from build123d import *

# Parameters (mm, degrees)
SKETCH_1_W          = 400
SKETCH_1_H          = 90
EXTRUDE_1_DEPTH     = 10
SKETCH_2_R          = 9.063152432
CUT_EXTRUDE_1_DEPTH = 10
SKETCH_3_R          = 1.81023823
SKETCH_3_R_2        = 1.954373085
SKETCH_3_R_3        = 2.399911157
SKETCH_3_R_4        = 2.359906839
CUT_EXTRUDE_2_DEPTH = 10
SKETCH_4_R          = 6.073356137
SKETCH_4_R_2        = 6.104859493
SKETCH_4_R_3        = 4.740379866
CUT_EXTRUDE_3_DEPTH = 10
SKETCH_5_W          = 12.49982796
SKETCH_5_H          = 90
EXTRUDE_2_DEPTH     = 270
SKETCH_6_W          = 148.075925294
SKETCH_6_H          = 90
CUT_EXTRUDE_4_DEPTH = 10
SKETCH_7_W          = 153.736310317
SKETCH_7_H          = 106.42917614
CUT_EXTRUDE_5_DEPTH = 10


with BuildPart() as part:
    # 草图1 → 凸台-拉伸1 (new body)
    with BuildSketch(Plane(origin=(0, 0, 0), x_dir=(1, 0, 0), z_dir=(0, 1, 0))):
        Rectangle(SKETCH_1_W, SKETCH_1_H)
    extrude(amount=EXTRUDE_1_DEPTH)

    # 草图2 → 切除-拉伸1 (cut)
    with BuildSketch(Plane(origin=(0, 10, 0), x_dir=(1, 0, 0), z_dir=(0, 1, 0))):
        with Locations((-6, 0)):
            Circle(SKETCH_2_R)
    extrude(amount=-CUT_EXTRUDE_1_DEPTH, mode=Mode.SUBTRACT)

    # 草图3 → 切除-拉伸2 (cut)
    with BuildSketch(Plane(origin=(0, 10, 0), x_dir=(1, 0, 0), z_dir=(0, 1, 0))):
        with Locations((-6, 25)):
            Circle(SKETCH_3_R)
        with Locations((19, 0)):
            Circle(SKETCH_3_R_2)
        with Locations((-6, -25)):
            Circle(SKETCH_3_R_3)
        with Locations((-31, 0)):
            Circle(SKETCH_3_R_4)
    extrude(amount=-CUT_EXTRUDE_2_DEPTH, mode=Mode.SUBTRACT)

    # 草图4 → 切除-拉伸3 (cut)
    with BuildSketch(Plane(origin=(0, 10, 0), x_dir=(1, 0, 0), z_dir=(0, 1, 0))):
        with Locations((-175, -21.552072621)):
            Circle(SKETCH_4_R)
        with Locations((-135, -21.552072621)):
            Circle(SKETCH_4_R_2)
        with Locations((-155, 23.447927379)):
            Circle(SKETCH_4_R_3)
    extrude(amount=-CUT_EXTRUDE_3_DEPTH, mode=Mode.SUBTRACT)

    # 草图5 → 凸台-拉伸2 (add)
    with BuildSketch(Plane(origin=(0, 10, 0), x_dir=(1, 0, 0), z_dir=(0, 1, 0))):
        with Locations((45.073880923, 0)):
            Rectangle(SKETCH_5_W, SKETCH_5_H)
    extrude(amount=EXTRUDE_2_DEPTH)

    # 草图6 → 切除-拉伸4 (cut)
    with BuildSketch(Plane.XZ):
        with Locations((-125.962037353, 0)):
            Rectangle(SKETCH_6_W, SKETCH_6_H)
    extrude(amount=-CUT_EXTRUDE_4_DEPTH, mode=Mode.SUBTRACT)

    # 草图7 → 切除-拉伸5 (cut)
    with BuildSketch(Plane(origin=(0, 10, 0), x_dir=(1, 0, 0), z_dir=(0, 1, 0))):
        with Locations((128.191950062, -8.21458807)):
            Rectangle(SKETCH_7_W, SKETCH_7_H)
    extrude(amount=-CUT_EXTRUDE_5_DEPTH, mode=Mode.SUBTRACT)


solid = part.part
Read the model definition and answer for the solid it produces. Units are mm, in the model's axes. A direction names the side the tool comes from. Coordinates: 2 decimals unless noted, no trailing zeros. Loops run counter-clockwise (first coordinate to the right, second up) from the corner with the lowest first, then second, coordinate; pieces in that order, holes last. Notation, with made-up numbers: (5, -8) -> (37, -8) arc R33 cw to (37, 27) -> close; hole circle Ø5 at (-33, -38.5). An arc over 180 degrees is marked (long way). Answer in a Markdown table with one row per item.
Item 1: A cutting plane is placed at C-C on y = 228. Determine the outline of the cut face in (x, z), plus the area to 3 significant figures.
Returned:
| item | result |
|---|---|
| outline | (38.82, -45) -> (51.32, -45) -> (51.32, 45) -> (38.82, 45) -> close |
| area | 1,120 mm^2 |
Item 2: Straight lines are drawn through the part: line 1 along Z through (x, y) = (-6, 4); line 2 along X through (y, z) = (8.25, 0); line 3 along Z through (x, y) = (-31, 2.5). For each, find the intervals that lie inside material, in ascending order. Write a range as [from, to].
Returned:
| item | result |
|---|---|
| line 1 | z = [-45, -26.81], [-23.19, -9.06], [9.06, 22.6], [27.4, 45] |
| line 2 | x = [-51.92, -33.36], [-28.64, -15.06], [3.06, 17.05], [20.95, 51.32] |
| line 3 | z = [-45, -2.36], [2.36, 45] |
Item 3: A cutting plane is placed at D-D on x = -22.5. Determine the outline of the cut face in (y, z).
Returned:
| item | result |
|---|---|
| outline | (0, -45) -> (10, -45) -> (10, 45) -> (0, 45) -> close |
Item 4: A cutting plane is placed at A-A on x = -11.5. Determine the outline of the cut face in (y, z).
Returned:
| item | result |
|---|---|
| outline | (0, -45) -> (10, -45) -> (10, -7.2) -> (0, -7.2) -> close; (0, 7.2) -> (10, 7.2) -> (10, 45) -> (0, 45) -> close |
Item 5: For faces 4 (the flat face through (38.824, 143, 1)), 5 (the flat face through (-1, 0, -11)), determine the directions among +Z, -Z, +X, -X, +Y, -Y from which every point of the face is accessible in a straight line to the end or side of a thin tool.
Returned:
| item | result |
|---|---|
| face 4 | +Z, -Z, -X, +Y |
| face 5 | +Z, -Z, +X, -X, -Y |
Item 6: For a pull along Z with two mould halves and no side action, classify faces 1 (the cylindrical face through (-12.68, 5.07, -6.125)), 2 (the flat face through (42, 108, -45)), 3 (the flat face through (45, 280, -1)) as released by +Z, released by -Z, zero draft, split by the parting line, or undercut.
Returned:
| item | result |
|---|---|
| face 1 | undercut |
| face 2 | released by -Z |
| face 3 | zero draft |
Item 7: A cutting plane is placed at B-B on z = 33. Determine the outline of the cut face in (x, y).
Returned:
| item | result |
|---|---|
| outline | (-51.92, 0) -> (51.32, 0) -> (51.32, 280) -> (38.82, 280) -> (38.82, 10) -> (-51.92, 10) -> close |
Item 8: Each of these flat-tipped pins is pushed along its axis until it touches: P1, Ø2, axis at x = 36, z = -18, coming from the +Y side; P2, Ø12, axis at y = 39.5, z = 4.5, coming from the -X side. Where does it stop, or does it pass through?
Returned:
| item | result |
|---|---|
| P1 | stops at y = 10 |
| P2 | stops at x = 38.82 |
